Part model, mm, in its own coordinate system. A direction names the side the tool comes from. Coordinates: 2 decimals unless noted, no trailing zeros. Loops run counter-clockwise (first coordinate to the right, second up) from the corner with the lowest first, then second, coordinate; pieces in that order, holes last. Notation, with made-up numbers: (67, -24) - (93, -24) arc R13 ccw to (93, -15) - close; hole circle Ø3 at (82.25, 10). An arc over 180 degrees is marked (long way). Use a Markdown table: item, result. Add a question column.
1. Wall check: probe 1 along Y at (x, z) = (3.75, 0); probe 2 along Y at (x, z) = (6.5, 0); probe 3 along X at (y, z) = (-2.5, -1.15). Give the ranges that are in metal, low to high. Write a range as [from, to].
2. Band-saw the part on B-B, the plane x = 6.75. Give the cut face in (y, z), plus the area to 3 significant figures.
3. Band-saw the part on A-A, the plane x = 4.25. Give the cut face in (y, z).
4. 3-axis set-ups, long thin cutter, end or side, ignore diameter. For faces 4 (the cylindrical face through (-4.76, -1.22, 0.27)), 5 (the cylindrical face through (0.07, -0.9, 2.86)), 6 (the cylindrical face through (6.4, -0.1, -2.5)): which of +Z, -Z, +X, -X, +Y, -Y reach the whole face in a straight line?
5. Drop flat-ended pins along their axis: pin 1 (1.5 mm diameter, centred on y = 0, z = 0, fed in from -X); pin 2 (1.5 mm diameter, centred on y = 2.5, z = -2.5, fed in from -X). Give the stop position or say it passes through.
6. Pull direction Y, two halves, no side cores. Call faces 1 (the cylindrical face through (-6.3, -0.1, -2.5)), 2 (the flat face through (7.8, 1, 1)), 3 (the conical face through (0.68, -0.21, 0.05)): pulls with the +Y half, pulls with the -Y half, needs draft (parallel to the pull), parting line crosses it, or undercut.
from build123d import *

# Parameters (mm, degrees)
HOLE_WIZARD_M3_2_D     = 2.5
HOLE_WIZARD_M3_2_DEPTH = 6
HOLE_WIZARD_M3_2_TIP   = 0.751075774
HOLE_WIZARD_M3_3_D     = 2.5
HOLE_WIZARD_M3_3_DEPTH = 6.5
HOLE_WIZARD_M3_3_TIP   = 0.751075774
CHAMFER_1_SIZE         = 0.1


with BuildPart() as part:
    # 草图2 → 旋转1 (revolve)
    with BuildSketch(Plane.XY, mode=Mode.PRIVATE) as revolve_1_sk:
        Polygon((-7.8, 0), (-7.8, 2.5), (-5, 2.5), (-5, 3), (5, 3), (5, 2.5), (7.8, 2.5), (7.8, 0), align=None)
    revolve(revolve_1_sk.sketch.rotate(Axis((-7.8, 0, 0), (1, 0, 0)), 90), axis=Axis((-7.8, 0, 0), (1, 0, 0)))

    # M3 螺纹孔2
    with Locations(Plane.ZY.offset(7.8)):
        with Locations((0, 0)):
            Hole(HOLE_WIZARD_M3_2_D / 2, depth=HOLE_WIZARD_M3_2_DEPTH)
            with Locations((0, 0, -(HOLE_WIZARD_M3_2_DEPTH + HOLE_WIZARD_M3_2_TIP / 2))):  # 118° drill point
                Cone(0, HOLE_WIZARD_M3_2_D / 2, HOLE_WIZARD_M3_2_TIP, mode=Mode.SUBTRACT)

    # M3 螺纹孔3
    with Locations(Plane(origin=(7.8, 0, 0), x_dir=(0, 0, -1), z_dir=(1, 0, 0))):
        with Locations((0, 0)):
            Hole(HOLE_WIZARD_M3_3_D / 2, depth=HOLE_WIZARD_M3_3_DEPTH)
            with Locations((0, 0, -(HOLE_WIZARD_M3_3_DEPTH + HOLE_WIZARD_M3_3_TIP / 2))):  # 118° drill point
                Cone(0, HOLE_WIZARD_M3_3_D / 2, HOLE_WIZARD_M3_3_TIP, mode=Mode.SUBTRACT)

    # 倒角1
    chamfer_1_edges = [part.edges().sort_by_distance(p)[0] for p in [
        (7.8, 0, -2.5),
        (5, 0, -3),
        (-5, 0, -3),
        (-7.8, 0, -2.5),
    ]]
    chamfer(chamfer_1_edges, length=CHAMFER_1_SIZE)


solid = part.part
Geometry check:
| question | item | result |
|---|---|---|
| 1 | probe 1 | y = [-3, -1.25], [1.25, 3] |
| 1 | probe 2 | y = [-2.5, -1.25], [1.25, 2.5] |
| 1 | probe 3 | x = [-5, 5] |
| 2 | outline | circle Ø5 at (0, 0); hole circle Ø2.5 at (0, 0) |
| 2 | area | 14.7 mm^2 |
| 3 | outline | circle Ø6 at (0, 0); hole circle Ø2.5 at (0, 0) |
| 4 | face 4 | -X |
| 4 | face 5 | +X, -X |
| 4 | face 6 | +X |
| 5 | pin 1 | stops at x = -1.5 |
| 5 | pin 2 | stops at x = -5 |
| 6 | face 1 | parting line crosses it |
| 6 | face 2 | needs draft |
| 6 | face 3 | undercut |
